```python
from build123d import *

# Parameters (mm, degrees)
F0_R     = 11.049
F1_DEPTH = 6.35


with BuildPart() as f1:
    # F0 (on Top) → F1 (new body)
    with BuildSketch(Plane.XY):
        with BuildLine():
            ThreePointArc((10.5094277958, -14.3415594481), (15.8585312405, -8.0396136036), (17.78, 0))
            ThreePointArc((17.78, 0), (15.6108797336, 8.5105131421), (9.6327745846, 14.9444991151))
            ThreePointArc((9.6327745846, 14.9444991151), (8.3729133787, 15.5596772314), (7.1654409141, 16.2722111745))
            ThreePointArc((7.1654409141, 16.2722111745), (-9.7140841192, 14.8917752376), (-17.78, 0))
            ThreePointArc((-17.78, 0), (-9.4273906442, -15.0749031719), (7.7827340428, -15.986164356))
            ThreePointArc((7.7827340428, -15.986164356), (9.1091896886, -15.102697614), (10.5094277958, -14.3415594481))
        make_face()
        Circle(F0_R, mode=Mode.SUBTRACT)
        with BuildLine():
            ThreePointArc((9.6327745846, 14.9444991151), (15.6108797336, 8.5105131421), (17.78, 0))
            ThreePointArc((17.78, 0), (15.8585312405, -8.0396136036), (10.5094277958, -14.3415594481))
            ThreePointArc((10.5094277958, -14.3415594481), (22.5963149024, -13.0765595999), (32.6723306155, -19.8711877644))
            ThreePointArc((32.6723306155, -19.8711877644), (30.024905988, 0.2187336146), (14.766870478, 13.5531308843))
            ThreePointArc((14.766870478, 13.5531308843), (12.1474957403, 14.0557311296), (9.6327745846, 14.9444991151))
        make_face()
        with BuildLine():
            ThreePointArc((14.766870478, 13.5531308843), (12.2321244934, 14.3680080122), (9.6327745846, 14.9444991151))
            ThreePointArc((9.6327745846, 14.9444991151), (12.1474957403, 14.0557311296), (14.766870478, 13.5531308843))
        make_face()
        with BuildLine():
            ThreePointArc((7.1654409141, 16.2722111745), (8.42530212, 15.6570330582), (9.6327745846, 14.9444991151))
            ThreePointArc((9.6327745846, 14.9444991151), (12.2321244934, 14.3680080122), (14.766870478, 13.5531308843))
            ThreePointArc((14.766870478, 13.5531308843), (28.6306092872, 17.9455815797), (34.5782154987, 31.2167102896))
            ThreePointArc((34.5782154987, 31.2167102896), (19.7525452394, 48.7495462206), (0, 37.0432320702))
            ThreePointArc((0, 37.0432320702), (-0.0097628586, 25.4184119581), (7.1654409141, 16.2722111745))
        make_face()
        with BuildLine():
            ThreePointArc((27.8472154987, 31.2167102896), (22.8348249156, 21.9625356777), (12.3454057878, 21.1046933455))
            ThreePointArc((12.3454057878, 21.1046933455), (10.7616060818, 40.4708849015), (27.8472154987, 31.2167102896))
        make_face(mode=Mode.SUBTRACT)
        with BuildLine():
            ThreePointArc((32.6723306155, -19.8711877644), (22.5963149024, -13.0765595999), (10.5094277958, -14.3415594481))
            ThreePointArc((10.5094277958, -14.3415594481), (9.1829721501, -15.2250261902), (7.7827340428, -15.986164356))
            ThreePointArc((7.7827340428, -15.986164356), (6.6242894769, -17.0632176818), (5.4082696447, -18.0748171313))
            ThreePointArc((5.4082696447, -18.0748171313), (11.6947079059, -46.8383870739), (36.0721618387, -30.3277238042))
            ThreePointArc((36.0721618387, -30.3277238042), (35.2008548818, -24.8300425135), (32.6723306155, -19.8711877644))
        make_face()
        with BuildLine():
            ThreePointArc((29.3411618387, -30.3277238042), (13.2961162421, -40.1826682179), (11.761303137, -21.4154690043))
            ThreePointArc((11.761303137, -21.4154690043), (23.2882074352, -20.4727793905), (29.3411618387, -30.3277238042))
        make_face(mode=Mode.SUBTRACT)
        with BuildLine():
            ThreePointArc((7.7827340428, -15.986164356), (9.1829721501, -15.2250261902), (10.5094277958, -14.3415594481))
            ThreePointArc((10.5094277958, -14.3415594481), (9.1091896886, -15.102697614), (7.7827340428, -15.986164356))
        make_face()
        with BuildLine():
            ThreePointArc((-17.78, 0), (-9.7140841192, 14.8917752376), (7.1654409141, 16.2722111745))
            ThreePointArc((7.1654409141, 16.2722111745), (-0.0097628586, 25.4184119581), (0, 37.0432320702))
            ThreePointArc((0, 37.0432320702), (-14.8117955692, 25.6039367366), (-19.4235623734, 7.4661757763))
            ThreePointArc((-19.4235623734, 7.4661757763), (-18.1957513695, 3.8224690318), (-17.78, 0))
        make_face()
        with BuildLine():
            ThreePointArc((5.4082696447, -18.0748171313), (6.5489734879, -16.9775954393), (7.7827340428, -15.986164356))
            ThreePointArc((7.7827340428, -15.986164356), (-9.4273906442, -15.0749031719), (-17.78, 0))
            ThreePointArc((-17.78, 0), (-21.5036758006, -10.8879819067), (-31.115, -17.2154109739))
            ThreePointArc((-31.115, -17.2154109739), (-13.0077535924, -24.206353637), (5.4082696447, -18.0748171313))
        make_face()
        with BuildLine():
            ThreePointArc((5.4082696447, -18.0748171313), (6.6242894769, -17.0632176818), (7.7827340428, -15.986164356))
            ThreePointArc((7.7827340428, -15.986164356), (6.5489734879, -16.9775954393), (5.4082696447, -18.0748171313))
        make_face()
        with BuildLine():
            ThreePointArc((-19.4235623734, 7.4661757763), (-18.851475509, 3.67812157), (-17.78, 0))
            ThreePointArc((-17.78, 0), (-18.1957513695, 3.8224690318), (-19.4235623734, 7.4661757763))
        make_face()
        with BuildLine():
            ThreePointArc((-31.115, -17.2154109739), (-21.5036758006, -10.8879819067), (-17.78, 0))
            ThreePointArc((-17.78, 0), (-18.851475509, 3.67812157), (-19.4235623734, 7.4661757763))
            ThreePointArc((-19.4235623734, 7.4661757763), (-51.6284185538, 7.6114601214), (-31.115, -17.2154109739))
        make_face()
        with Locations((-35.56, 0)):
            Circle(F0_R, mode=Mode.SUBTRACT)
    extrude(amount=F1_DEPTH)


solid = f1.part
```
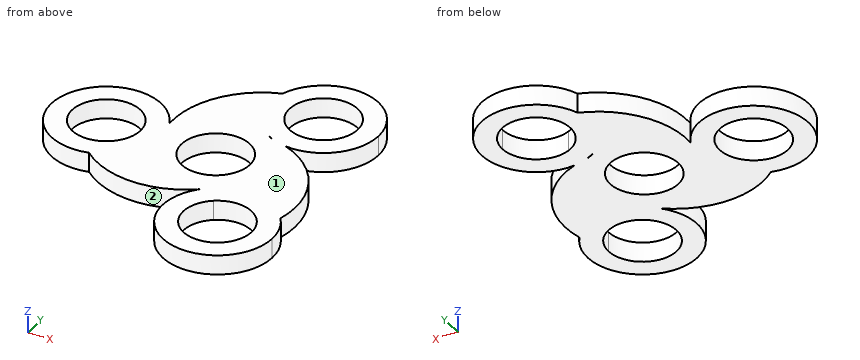
Can you work these out from the model? Positions are in its coordinate system, mm. Face numbers are marked on the shaded views. Round coordinates to 2 decimals unless told otherwise and drop trailing zeros. Loops run counter-clockwise (first coordinate to the right, second up) from the corner with the lowest first, then second, coordinate; pieces in that order, holes last. Notation, with made-up numbers: M -25.5,-24.5 L -10.5,-24.5 A26 cw -10.5,0.5 Z; hole C 66,60 d7. An arc over 180 degrees is marked long. Answer as a JSON object with one key per item and string values. Group by question number.
Q1. Imagine slicing it at B-B, the plane z = 2.5. Please give me the cut outline in (x, y) (1 decimal).
Q2. Imagine slicing it at D-D, the plane y = -22.5. Please give me the cut outline in (x, z), then the cut area to 3 significant figures.
Q3. Imagine slicing it at A-A, the plane x = -35.56. Please give me the cut outline in (y, z).
Q4. Imagine slicing it at C-C, the plane y = 2. Please give me the cut outline in (x, z).
Q5. Will these pins go through, and if not, where does the flat tip stop? pin 1 (3 mm diameter, centred on x = 14.5, z = 2, fed in from +Y); pin 2 (3 mm diameter, centred on x = -26, z = 1.5, fed in from +Y); pin 3 (1.5 mm diameter, centred on x = 26.5, y = 28.5, fed in from +Z).
Q6. Please list where these lines run through material, in increasing order: L1, parallel to Y at x = 16.5, z = 2.5; L2, parallel to X at y = -5, z = 4; L3, parallel to Y at x = 3.5, z = 3.25.
Q7. We'd pull the mould along X, two halves only. Please class the marked faces 1 and 2: +X half, -X half, draft (parallel to the pull), parting line (faces both ways), or undercut.
Findings:
{
 "1": {"outline": "M -31.1,-17.2 A28.7 ccw 5.4,-18.1 A17.8 ccw long 32.7,-19.9 A28.7 ccw 14.8,13.6 A17.8 ccw long 0,37 A28.7 ccw -19.4,7.5 A17.8 ccw long Z; hole C -35.6,0 d22.1; hole C 0,0 d22.1; hole C 16.8,31.2 d22.1; hole C 18.3,-30.3 d22.1; hole M 7.2,16.3 A17.8 ccw 9.6,14.9 A17.8 ccw Z"},
 "2": {"outline": "M -22.1,0 L -2.56,0 L -2.56,6.35 L -22.1,6.35 Z; M 2.33,0 L 10.49,0 L 10.49,6.35 L 2.33,6.35 Z; M 26.09,0 L 34.26,0 L 34.26,6.35 L 26.09,6.35 Z", "area": "228 mm2"},
 "3": {"outline": "M -17.78,0 L -11.05,0 L -11.05,6.35 L -17.78,6.35 Z; M 11.05,0 L 17.78,0 L 17.78,6.35 L 11.05,6.35 Z"},
 "4": {"outline": "M -53.23,0 L -46.43,0 L -46.43,6.35 L -53.23,6.35 Z; M -24.69,0 L -10.87,0 L -10.87,6.35 L -24.69,6.35 Z; M 10.87,0 L 28.99,0 L 28.99,6.35 L 10.87,6.35 Z"},
 "5": {"pin 1": "stops at y = 48.98", "pin 2": "stops at y = 15.85", "pin 3": "passes through"},
 "6": {"L1": "y = -48.02 to -41.23, -19.43 to 12.84, 13.44 to 20.17, 42.26 to 48.99", "L2": "x = -52.62 to -45.41, -25.71 to -9.85, 9.85 to 32.19", "L3": "y = -40.19 to -20.46, -19.45 to -10.48, 10.48 to 43.02"},
 "7": {"face 1": "draft", "face 2": "undercut"}
}
